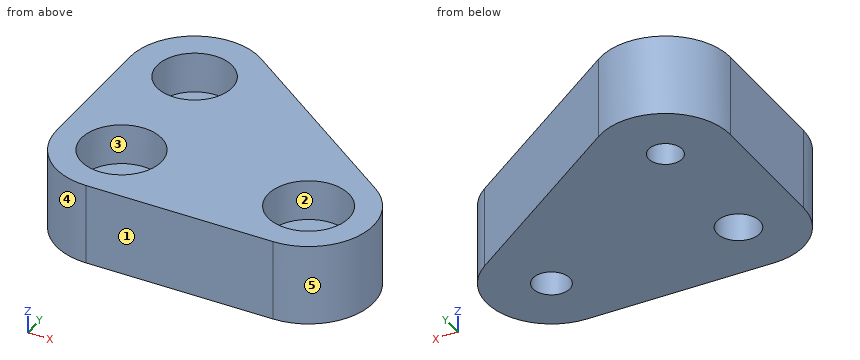
from build123d import *

# Parameters (mm, degrees)
F0_R     = 9.852424
F0_R_2   = 9.947133
F0_R_3   = 9.245087
F1_DEPTH = 20
F0_R_4   = 4.115098
F0_R_5   = 5.263248
F0_R_6   = 4.528776
F2_DEPTH = 10


with BuildPart() as f1:
    # F0 (on Top) → F1 (new body)
    with BuildSketch(Plane.XY):
        with BuildLine():
            ThreePointArc((0, 16), (4.686292, 4.686292), (16, 0))
            Line((16, 0), (62.072559, 0))
            ThreePointArc((62.072559, 0), (77.309287, 11.117161), (71.37237, 29.019736))
            Line((71.37237, 29.019736), (25.299811, 61.928706))
            ThreePointArc((25.299811, 61.928706), (8.678695, 63.135653), (0, 48.908971))
            Line((0, 48.908971), (0, 16))
        make_face()
        with Locations((16, 16)):
            Circle(F0_R, mode=Mode.SUBTRACT)
        with Locations((62.072559, 16)):
            Circle(F0_R_2, mode=Mode.SUBTRACT)
        with Locations((16, 48.908971)):
            Circle(F0_R_3, mode=Mode.SUBTRACT)
    extrude(amount=F1_DEPTH)

    # F0 (on Top) → F2 (join)
    with BuildSketch(Plane.XY):
        with BuildLine():
            ThreePointArc((0, 16), (4.686292, 4.686292), (16, 0))
            Line((16, 0), (62.072559, 0))
            ThreePointArc((62.072559, 0), (77.309287, 11.117161), (71.37237, 29.019736))
            Line((71.37237, 29.019736), (25.299811, 61.928706))
            ThreePointArc((25.299811, 61.928706), (8.678695, 63.135653), (0, 48.908971))
            Line((0, 48.908971), (0, 16))
        make_face()
        with Locations((16, 16)):
            Circle(F0_R, mode=Mode.SUBTRACT)
        with Locations((62.072559, 16)):
            Circle(F0_R_2, mode=Mode.SUBTRACT)
        with Locations((16, 48.908971)):
            Circle(F0_R_3, mode=Mode.SUBTRACT)
        with Locations((16, 48.908971)):
            Circle(F0_R_3)
        with Locations((16, 48.908971)):
            Circle(F0_R_4, mode=Mode.SUBTRACT)
        with Locations((16, 16)):
            Circle(F0_R)
        with Locations((16, 16)):
            Circle(F0_R_5, mode=Mode.SUBTRACT)
        with Locations((62.072559, 16)):
            Circle(F0_R_2)
        with Locations((62.072559, 16)):
            Circle(F0_R_6, mode=Mode.SUBTRACT)
    extrude(amount=F2_DEPTH)


solid = f1.part
Read the model definition and answer for the solid it produces. Units are mm, in the model's axes. Face numbers are marked on the shaded views. A direction names the side the tool comes from. Give positions to 0.01 mm unless a question says otherwise; leave off trailing zeros. Loops run counter-clockwise (first coordinate to the right, second up) from the corner with the lowest first, then second, coordinate; pieces in that order, holes last. Notation, with made-up numbers: (24, 48) -> (43, 48) arc R21 cw to (43, 52) -> close; hole circle Ø5 at (-10.5, -21). An arc over 180 degrees is marked (long way). Answer as CSV lines item,"result".
Item 1: Find section D-D on y = 7.5. Give the vertices of the cut face in (x, z), plus the area to 3 significant figures.
Returned:
outline,"(2.44, 0) -> (75.63, 0) -> (75.63, 20) -> (67.24, 20) -> (67.24, 10) -> (56.91, 10) -> (56.91, 20) -> (20.98, 20) -> (20.98, 10) -> (11.02, 10) -> (11.02, 20) -> (2.44, 20) -> close"
area,"1,260 mm²"
Item 2: Find section C-C on z = 6. Give the vertices of the cut face in (x, y).
Returned:
outline,"(0, 16) arc R16 ccw to (16, 0) -> (62.07, 0) arc R16 ccw to (71.37, 29.02) -> (25.3, 61.93) arc R16 ccw to (0, 48.91) -> close; hole circle Ø10.53 at (16, 16); hole circle Ø8.23 at (16, 48.91); hole circle Ø9.06 at (62.07, 16)"
Item 3: Find section B-B on x = 69.5. Give the vertices of the cut face in (y, z), plus the area to 3 significant figures.
Returned:
outline,"(1.83, 0) -> (30.36, 0) -> (30.36, 20) -> (22.62, 20) -> (22.62, 10) -> (9.38, 10) -> (9.38, 20) -> (1.83, 20) -> close"
area,"438 mm²"
Item 4: Consider line 1 (X direction, y = 16, z = 13.25); line 2 (Y direction, x = 16, z = 6.25); line 3 (Y direction, x = 14, z = 5.5). Determine where each line is inside the solid, lowest interval first. Write a range as [from, to].
Returned:
line 1,"x = [0, 6.15], [25.85, 52.13], [72.02, 78.07]"
line 2,"y = [0, 10.74], [21.26, 44.79], [53.02, 64.91]"
line 3,"y = [0.13, 11.13], [20.87, 45.31], [52.51, 64.78]"
Item 5: Find section A-A on z = 17. Give the vertices of the cut face in (x, y).
Returned:
outline,"(0, 16) arc R16 ccw to (16, 0) -> (62.07, 0) arc R16 ccw to (71.37, 29.02) -> (25.3, 61.93) arc R16 ccw to (0, 48.91) -> close; hole circle Ø19.7 at (16, 16); hole circle Ø18.49 at (16, 48.91); hole circle Ø19.89 at (62.07, 16)"
Item 6: Determine the mould class of the marked faces 3, 4 and 5 for opening direction X: +X half, -X half, draft (parallel to the pull), parting line (faces both ways), or undercut.
Returned:
face 3,"undercut"
face 4,"-X half"
face 5,"+X half"
Item 7: For the marked faces 1 and 2, determine the directions among +Z, -Z, +X, -X, +Y, -Y from which every point of the face is accessible in a straight line to the end or side of a thin tool.
Returned:
face 1,"+Z, -Z, +X, -X, -Y"
face 2,"+Z"
Item 8: Each of these flat-tipped pins is pushed along its axis until it touches: pin 1 (9.5 mm diameter, centred on x = 16, y = 48.91, fed in from +Z); pin 2 (4 mm diameter, centred on y = 57, z = 14, fed in from +X); pin 3 (8 mm diameter, centred on y = 11, z = 3.5, fed in from +X); pin 4 (8.5 mm diameter, centred on x = 16, y = 16, fed in from +Z). Where does it stop, or does it pass through?
Returned:
pin 1,"stops at z = 10"
pin 2,"stops at x = 35"
pin 3,"stops at x = 78.04"
pin 4,"passes through"
